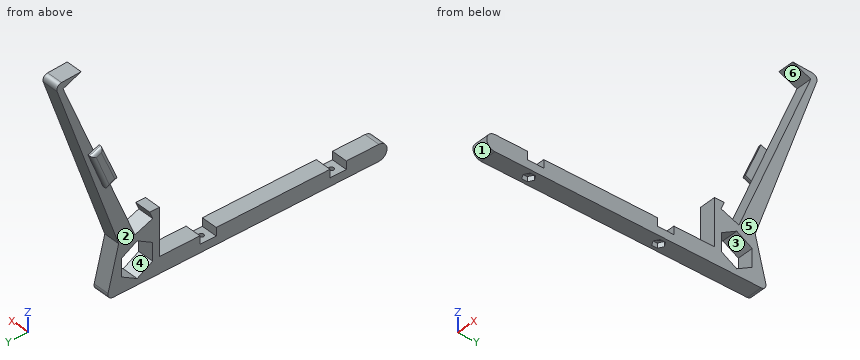
from build123d import *

# Parameters (mm, degrees)
PAD_DEPTH       = 10
SKETCH001_R     = 1.5
POCKET_DEPTH    = 5
PAD001_DEPTH    = 3
FILLET_R        = 2
FILLET001_R     = 3
FILLET002_R     = 3
POCKET001_DEPTH = 3


with BuildPart() as part:
    # Sketch → Pad (new body)
    with BuildSketch(Plane.YZ):
        with BuildLine():
            Line((33.085568, 111.431625), (44.200844, 106.790084))
            Line((44.200844, 106.790084), (0, 0))
            Line((0, 0), (-10.926105, 4.190362))
            Line((-10.926105, 4.190362), (-9.043063, 8.84724))
            Line((-9.043063, 8.84724), (-15, 8.84724))
            Line((-15, 8.84724), (-15, -20))
            Line((-15, -20), (-40, -20))
            Line((-40, -25), (-40, -20))
            Line((-50, -25), (-40, -25))
            Line((-50, -20), (-50, -25))
            Line((-50, -20), (-120, -20))
            Line((-120, -25), (-120, -20))
            Line((-130, -25), (-120, -25))
            Line((-130, -20), (-130, -25))
            Line((-130, -20), (-150, -20))
            ThreePointArc((-150, -20), (-155, -25), (-150, -30))
            Line((-150, -30), (17.484663, -30))
            Line((17.484663, -30), (10, -0.272781))
            Line((10, -0.272781), (49.18668, 110.743774))
            Line((49.18668, 110.743774), (33.085568, 111.431625))
        make_face()
        Polygon((8.178281, -20.684753), (8.178281, -9.690605), (-1.342931, -4.193531), (-10.864143, -9.690605), (-10.864143, -20.684753), (-1.342931, -26.181827), align=None, mode=Mode.SUBTRACT)
    extrude(amount=PAD_DEPTH)

    # Sketch001 → Pocket (cut)
    with BuildSketch(Plane(origin=(0, 0, -25), x_dir=(0, -1, 0), z_dir=(0, 0, 1))):
        with Locations((45, 5)):
            Circle(SKETCH001_R)
        with Locations((125, 5)):
            Circle(SKETCH001_R)
    extrude(amount=-POCKET_DEPTH, mode=Mode.SUBTRACT)

    # Sketch003 → Pad001 (new body)
    with BuildSketch(Plane(origin=(0, 0, 0), x_dir=(0, 1, 0), z_dir=(-1, 0, 0))):
        Polygon((19.571926, -37.694836), (28.872379, -60.69595), (22.072046, -63.396084), (12.471581, -40.894993), align=None)
    extrude(amount=PAD001_DEPTH)

    # Fillet
    fillet_edges = [part.edges().sort_by_distance(p)[0] for p in [
        (-3, 24.222153, 49.195393),
        (-3, 25.472213, 62.046017),
        (-3, 17.271813, 52.145538),
        (-3, 16.021754, 39.294915),
    ]]
    fillet(fillet_edges, radius=FILLET_R)

    # Fillet001
    fillet001_edges = [part.edges().sort_by_distance(p)[0] for p in [
        (5, 49.18668, 110.743774),
    ]]
    fillet(fillet001_edges, radius=FILLET001_R)

    # Fillet002
    fillet002_edges = [part.edges().sort_by_distance(p)[0] for p in [
        (5, 17.484663, -30),
    ]]
    fillet(fillet002_edges, radius=FILLET002_R)

    # Sketch002 → Pocket001 (cut)
    with BuildSketch(Plane.YX.offset(30)):
        Polygon((-123.239415, 1.964181), (-121.507364, 4.964181), (-123.239415, 7.964181), (-126.703517, 7.964181), (-128.435568, 4.964181), (-126.703517, 1.964181), align=None)
        Polygon((-43.334626, 7.980642), (-46.798728, 7.980642), (-48.530779, 4.980642), (-46.798728, 1.980642), (-43.334626, 1.980642), (-41.602575, 4.980642), align=None)
    extrude(amount=-POCKET001_DEPTH, mode=Mode.SUBTRACT)


solid = part.part
Geometry check sheet. Reference: the model listing, model coordinates, mm. Face numbers are marked on the shaded views. A direction names the side the tool comes from. Coordinates: 2 decimals unless noted, no trailing zeros. Order: outer loops, then holes, each group sorted by start corner. A loop starts at its lowest first (then second) coordinate and runs counter-clockwise, first axis right, second up. Notation, with made-up numbers: (65, -2) - (99, -2) arc R21 cw to (99, 10) - close; hole circle Ø3 at (36, 64.5). An arc over 180 degrees is marked (long way). Answer in a Markdown table with one row per item. Add a question column.
1) Gauge pin test, flat ends, axial feed: P1, Ø5.5, axis at x = 5.5, z = -22, coming from the -Y side; P2, Ø4, axis at x = 3.5, z = -22, coming from the +Y side; P3, Ø1.8, axis at x = 4, y = -123.5, coming from the -Z side; P4, Ø1.8, axis at x = 5, y = -45, coming from the -Z side. Record the tip position at first contact, or that the pin passes through.
2) Cross-section at A-A, the plane y = -63. Record the cut outline in (x, z).
3) Cross-section at B-B, the plane z = 11. Record the cut outline in (x, y), then the cut area to 3 significant figures.
4) Set-up check for the marked faces 5 and 6: record each of +Z, -Z, +X, -X, +Y, -Y from which the full face is reachable in a straight line by a thin tool's end or side.
5) Material ranges on line 1 along X through (y, z) = (-45, -25.95); line 2 along Z through (x, y) = (9, -55.5); line 3 along Y through (x, z) = (0.5, -22.5), recorded low to high. Write a range as [from, to].
6) Release check for a two-part mould opening along Z. For the marked faces 1, 2, 3 and 4 record: +Z half, -Z half, draft (parallel to the pull), parting line (faces both ways), or undercut.
Check result:
| question | item | result |
|---|---|---|
| 1 | P1 | stops at y = -154.99 |
| 1 | P2 | stops at y = 15.97 |
| 1 | P3 | stops at z = -27 |
| 1 | P4 | passes through |
| 2 | outline | (0, -30) - (10, -30) - (10, -20) - (0, -20) - close |
| 3 | outline | (0, 4.55) - (10, 4.55) - (10, 13.98) - (0, 13.98) - close |
| 3 | area | 94.3 mm² |
| 4 | face 5 | +Z, -Z, +X, +Y, -Y |
| 4 | face 6 | +X, -X, -Y |
| 5 | line 1 | x = [0, 3.5], [6.5, 10] |
| 5 | line 2 | z = [-30, -20] |
| 5 | line 3 | y = [-154.33, -130], [-120, -50], [-40, -7.72], [5.03, 15.6] |
| 6 | face 1 | parting line |
| 6 | face 2 | draft |
| 6 | face 3 | undercut |
| 6 | face 4 | undercut |
